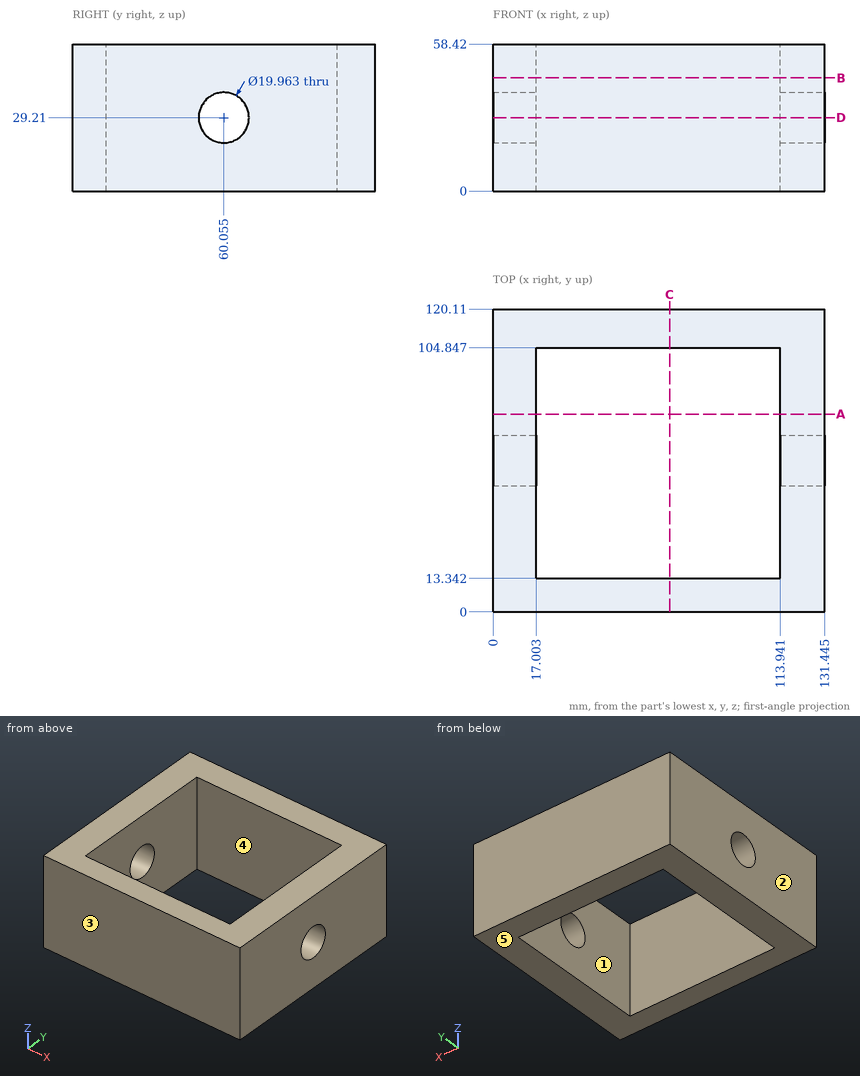
Study the drawing (mm; zero at the part's minimum x, y, z) and answer. A direction names the side the tool comes from. Give positions to 0.01 mm unless a question says otherwise; leave off trailing zeros. Write each loop counter-clockwise with the first axis right and the second up, starting at its lowest first coordinate (ties: lowest second). Pieces come first, ordered by that corner, then holes. Notation, with made-up numbers: M 23.25,71 L 49.25,71 A32 cw 49.25,97 Z; hole C 1.5,70 d11. An arc over 180 degrees is marked long. Put each result on its own line as item: value. Start each with the question number.
1. For a pull along Y with two mould halves and no side action, classify the marked faces 1, 2 and 3 as released by +Y, released by -Y, zero draft, split by the parting line, or undercut.
2. Consider line 1 along Y through (x, z) = (76, 41); line 2 along X through (y, z) = (18.5, 27.5) (1 decimal); line 3 along Y through (x, z) = (11, 29) (1 decimal). Determine where each line is inside the solid, lowest interval first.
3. Each of these flat-tipped pins is pushed along its axis until it touches: pin 1 Ø1.5 at (y, z) = (16.5, 39) entering from -X; pin 2 Ø12 at (y, z) = (60.06, 29.21) entering from +X. Where does it stop, or does it pass through?
4. Which of the six approach directions +Z, -Z, +X, -X, +Y, -Y give full straight-line access (tool end or side, diameter ignored) to the marked faces 4 and 5?
5. The part is cut by section B-B, the plane z = 45. Give the vertices of the cut face in (x, y) (1 decimal), and give its area (3 significant figures).
6. The part is cut by section C-C, the plane x = 70. Give the vertices of the cut face in (y, z), and give its area (3 significant figures).
7. The part is cut by section A-A, the plane y = 78.5. Give the vertices of the cut face in (x, z) (1 decimal).
8. The part is cut by section D-D, the plane z = 29.21. Give the vertices of the cut face in (x, y) (1 decimal), and give its area (3 significant figures).
Final values:
1. face 1: undercut
1. face 2: zero draft
1. face 3: released by -Y
2. line 1: y = 0 to 13.34, 104.85 to 120.11
2. line 2: x = 0 to 17, 113.9 to 131.4
2. line 3: y = 0 to 50.1, 70 to 120.1
3. pin 1: stops at x = 0
3. pin 2: passes through
4. face 4: +Z, -Z
4. face 5: -Z, +X, -X, +Y, -Y
5. outline: M 0,0 L 131.4,0 L 131.4,120.1 L 0,120.1 Z; hole M 17,13.3 L 113.9,13.3 L 113.9,104.8 L 17,104.8 Z
5. area: 6,920 mm²
6. outline: M 0,0 L 13.34,0 L 13.34,58.42 L 0,58.42 Z; M 104.85,0 L 120.11,0 L 120.11,58.42 L 104.85,58.42 Z
6. area: 1,670 mm²
7. outline: M 0,0 L 17,0 L 17,58.4 L 0,58.4 Z; M 113.9,0 L 131.4,0 L 131.4,58.4 L 113.9,58.4 Z
8. outline: M 0,0 L 131.4,0 L 131.4,50.1 L 113.9,50.1 L 113.9,13.3 L 17,13.3 L 17,50.1 L 0,50.1 Z; M 0,70 L 17,70 L 17,104.8 L 113.9,104.8 L 113.9,70 L 131.4,70 L 131.4,120.1 L 0,120.1 Z
8. area: 6,230 mm²
